from build123d import *

# Parameters (mm, degrees)
SKETCH1_W           = 76.33
SKETCH1_H           = 76.33
BOSS_EXTRUDE1_DEPTH = 76.33
SKETCH2_R           = 35
BOSS_EXTRUDE2_DEPTH = 36.82
CHAMFER1_SIZE       = 2.5
CUT_EXTRUDE1_REACH  = 1889.491
CUT_EXTRUDE2_DEPTH  = 0.5


with BuildPart() as part:
    # Sketch1 → Boss-Extrude1 (new body)
    with BuildSketch(Plane.ZY.offset(-1848.740517551)):
        Rectangle(SKETCH1_W, SKETCH1_H)
    extrude(amount=BOSS_EXTRUDE1_DEPTH)

    # Sketch2 → Boss-Extrude2 (add)
    with BuildSketch(Plane(origin=(1848.740517551, 0, 0), x_dir=(0, 0, -1), z_dir=(1, 0, 0))):
        with Locations(Location((0, 0, 0), (0, 0, 90))):
            Circle(SKETCH2_R)
    extrude(amount=BOSS_EXTRUDE2_DEPTH)

    # Chamfer1
    chamfer1_edges = [part.edges().sort_by_distance(p)[0] for p in [
        (1772.410517551, -38.165, 0),
        (1772.410517551, 0, -38.165),
        (1772.410517551, 38.165, 0),
        (1848.740517551, 0, -38.165),
        (1848.740517551, -38.165, 0),
        (1848.740517551, 0, 38.165),
        (1848.740517551, 38.165, 0),
        (1772.410517551, 0, 38.165),
        (1810.575517551, 38.165, -38.165),
        (1810.575517551, -38.165, -38.165),
        (1810.575517551, -38.165, 38.165),
        (1810.575517551, 38.165, 38.165),
    ]]
    chamfer(chamfer1_edges, length=CHAMFER1_SIZE)

    # Sketch3 → Cut-Extrude1 (cut, up to next)
    with BuildSketch(Plane(origin=(0, 0, -38.165), x_dir=(-1, 0, 0), z_dir=(0, 0, -1)), mode=Mode.PRIVATE) as cut_extrude1_sk1:
        with BuildLine():
            ThreePointArc((-1791.865517551, 0), (-1797.345549675, 13.229967876), (-1810.575517551, 18.71))
            Line((-1810.575517551, 18.71), (-1810.575517551, -18.71))
            ThreePointArc((-1810.575517551, -18.71), (-1797.345549675, -13.229967876), (-1791.865517551, 0))
        make_face()
    cut_extrude1_tool1 = extrude(cut_extrude1_sk1.sketch, amount=-CUT_EXTRUDE1_REACH, mode=Mode.PRIVATE) & part.part
    # Sketch3 → Cut-Extrude1 (cut, up to next)
    with BuildSketch(Plane(origin=(0, 0, -38.165), x_dir=(-1, 0, 0), z_dir=(0, 0, -1)), mode=Mode.PRIVATE) as cut_extrude1_sk2:
        with BuildLine():
            Line((-1810.575517551, -18.71), (-1810.575517551, 18.71))
            ThreePointArc((-1810.575517551, 18.71), (-1829.285517551, 0), (-1810.575517551, -18.71))
        make_face()
    cut_extrude1_tool2 = extrude(cut_extrude1_sk2.sketch, amount=-CUT_EXTRUDE1_REACH, mode=Mode.PRIVATE) & part.part
    # Sketch3 → Cut-Extrude1 (cut, up to next)
    with BuildSketch(Plane(origin=(0, 0, -38.165), x_dir=(-1, 0, 0), z_dir=(0, 0, -1)), mode=Mode.PRIVATE) as cut_extrude1_sk3:
        with BuildLine():
            ThreePointArc((-1791.865517551, 0), (-1797.345549675, 13.229967876), (-1810.575517551, 18.71))
            Line((-1810.575517551, 18.71), (-1810.575517551, -18.71))
            ThreePointArc((-1810.575517551, -18.71), (-1797.345549675, -13.229967876), (-1791.865517551, 0))
        make_face()
    cut_extrude1_tool3 = extrude(cut_extrude1_sk3.sketch, amount=-CUT_EXTRUDE1_REACH, mode=Mode.PRIVATE) & part.part
    # Sketch3 → Cut-Extrude1 (cut, up to next)
    with BuildSketch(Plane(origin=(0, 0, -38.165), x_dir=(-1, 0, 0), z_dir=(0, 0, -1)), mode=Mode.PRIVATE) as cut_extrude1_sk4:
        with BuildLine():
            Line((-1810.575517551, -18.71), (-1810.575517551, 18.71))
            ThreePointArc((-1810.575517551, 18.71), (-1829.285517551, 0), (-1810.575517551, -18.71))
        make_face()
    cut_extrude1_tool4 = extrude(cut_extrude1_sk4.sketch, amount=-CUT_EXTRUDE1_REACH, mode=Mode.PRIVATE) & part.part
    add(cut_extrude1_tool1.solids().sort_by_distance((1802.634747, 0, -38.165))[0], mode=Mode.SUBTRACT)
    add(cut_extrude1_tool2.solids().sort_by_distance((1818.516288, 0, -38.165))[0], mode=Mode.SUBTRACT)
    add(cut_extrude1_tool3.solids().sort_by_distance((1802.634747, 0, -38.165))[0], mode=Mode.SUBTRACT)
    add(cut_extrude1_tool4.solids().sort_by_distance((1818.516288, 0, -38.165))[0], mode=Mode.SUBTRACT)

    # Sketch5 → Cut-Extrude2 (cut)
    with BuildSketch(Plane(origin=(0, 38.165, 0), x_dir=(1, 0, 0), z_dir=(0, 1, 0))):
        with BuildLine():
            Line((1788.358917551, -32.3946), (1832.792217551, -32.3946))
            add(Edge.make_bspline(
                [(1832.792217551, -32.3946), (1833.466855861, -32.3946), (1834.834608919, -32.253703608), (1837.339344692, -31.462150857), (1840.043615022, -29.624585418), (1841.881171353, -26.92029094), (1842.672721425, -24.415524634), (1842.813617551, -23.047748692), (1842.813617551, -22.3731)],
                knots=[0.555555556, 0.555555556, 0.555555556, 0.555555556, 0.569444444, 0.583333333, 0.611111111, 0.638888889, 0.652777778, 0.666666667, 0.666666667, 0.666666667, 0.666666667], degree=3))
            Line((1842.813617551, -22.3731), (1842.813617551, 22.373))
            add(Edge.make_bspline(
                [(1842.813617551, 22.373), (1842.813617551, 23.047629093), (1842.672720901, 24.415360154), (1841.881169744, 26.92007933), (1840.043614741, 29.624353237), (1837.339347144, 31.46193401), (1834.834610984, 32.25350014), (1833.466856595, 32.3944), (1832.792217551, 32.3944)],
                knots=[0.777777778, 0.777777778, 0.777777778, 0.777777778, 0.805555556, 0.833333333, 0.888888889, 0.944444444, 0.972222222, 1, 1, 1, 1], degree=3))
            Line((1832.792217551, 32.3944), (1788.358917551, 32.3944))
            add(Edge.make_bspline(
                [(1788.358917551, 32.3944), (1787.684278508, 32.3944), (1786.316524118, 32.25350014), (1783.811787958, 31.46193401), (1781.107520362, 29.624353237), (1779.269965358, 26.92007933), (1778.478414202, 24.415360154), (1778.337517551, 23.047629093), (1778.337517551, 22.373)],
                knots=[0.111111111, 0.111111111, 0.111111111, 0.111111111, 0.125, 0.138888889, 0.166666667, 0.194444444, 0.208333333, 0.222222222, 0.222222222, 0.222222222, 0.222222222], degree=3))
            Line((1778.337517551, 22.373), (1778.337517551, -22.3731))
            add(Edge.make_bspline(
                [(1778.337517551, -22.3731), (1778.337517551, -23.047748692), (1778.478413677, -24.415524634), (1779.269963749, -26.92029094), (1781.107520081, -29.624585418), (1783.81179041, -31.462150857), (1786.316526183, -32.253703608), (1787.684279242, -32.3946), (1788.358917551, -32.3946)],
                knots=[0.333333333, 0.333333333, 0.333333333, 0.333333333, 0.347222222, 0.361111111, 0.388888889, 0.416666667, 0.430555556, 0.444444444, 0.444444444, 0.444444444, 0.444444444], degree=3))
        make_face()
        with BuildLine():
            Line((1788.358917551, -31.3946), (1832.792217551, -31.3946))
            add(Edge.make_bspline(
                [(1832.792217551, -31.3946), (1833.399248628, -31.3946), (1834.630365029, -31.267771469), (1836.881569909, -30.556358134), (1839.319622864, -28.900598899), (1840.975375901, -26.462522118), (1841.686788747, -24.211284373), (1841.813617551, -22.980142574), (1841.813617551, -22.3731)],
                knots=[0.555555556, 0.555555556, 0.555555556, 0.555555556, 0.569444444, 0.583333333, 0.611111111, 0.638888889, 0.652777778, 0.666666667, 0.666666667, 0.666666667, 0.666666667], degree=3))
            Line((1841.813617551, -22.3731), (1841.813617551, 22.373))
            add(Edge.make_bspline(
                [(1841.813617551, 22.373), (1841.813617551, 22.980021237), (1841.686789271, 24.211113504), (1840.975377513, 26.462304848), (1839.319623121, 28.900367756), (1836.881567526, 30.556143835), (1834.630362845, 31.267568666), (1833.399248157, 31.3944), (1832.792217551, 31.3944)],
                knots=[0.777777778, 0.777777778, 0.777777778, 0.777777778, 0.805555556, 0.833333333, 0.888888889, 0.944444444, 0.972222222, 1, 1, 1, 1], degree=3))
            Line((1832.792217551, 31.3944), (1788.358917551, 31.3944))
            add(Edge.make_bspline(
                [(1788.358917551, 31.3944), (1787.751886946, 31.3944), (1786.520772257, 31.267568666), (1784.269567577, 30.556143835), (1781.831511982, 28.900367756), (1780.175757589, 26.462304848), (1779.464345832, 24.211113504), (1779.337517551, 22.980021237), (1779.337517551, 22.373)],
                knots=[0.111111111, 0.111111111, 0.111111111, 0.111111111, 0.125, 0.138888889, 0.166666667, 0.194444444, 0.208333333, 0.222222222, 0.222222222, 0.222222222, 0.222222222], degree=3))
            Line((1779.337517551, 22.373), (1779.337517551, -22.3731))
            add(Edge.make_bspline(
                [(1779.337517551, -22.3731), (1779.337517551, -22.980142574), (1779.464346356, -24.211284373), (1780.175759201, -26.462522118), (1781.831512239, -28.900598899), (1784.269565194, -30.556358134), (1786.520770074, -31.267771469), (1787.751886474, -31.3946), (1788.358917551, -31.3946)],
                knots=[0.333333333, 0.333333333, 0.333333333, 0.333333333, 0.347222222, 0.361111111, 0.388888889, 0.416666667, 0.430555556, 0.444444444, 0.444444444, 0.444444444, 0.444444444], degree=3))
        make_face(mode=Mode.SUBTRACT)
    extrude(amount=-CUT_EXTRUDE2_DEPTH, mode=Mode.SUBTRACT)


solid = part.part
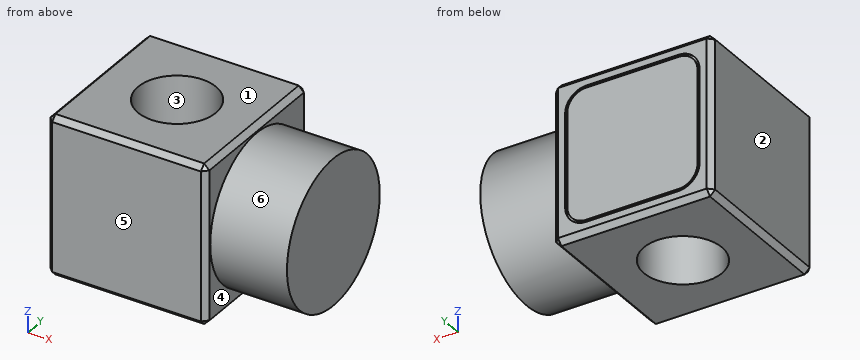
Here's how the part is built. I have some questions about the finished solid (model axes, mm). Face numbers are marked on the shaded views. A direction names the side the tool comes from. Round coordinates to 2 decimals unless told otherwise and drop trailing zeros. Write each loop counter-clockwise with the first axis right and the second up, starting at its lowest first coordinate (ties: lowest second). Pieces come first, ordered by that corner, then holes. Notation, with made-up numbers: (54.25, 49) -> (69.25, 49) arc R22 cw to (69.25, 69) -> close; hole circle Ø9 at (-15, 16.5). An arc over 180 degrees is marked (long way). One line per item, written item: value.
1) Suppose I cut it at C-C on x = 1800. List the corners of the cut face in (y, z) for me (3 decimals).
Filled sheet:
outline: (-38.165, -35.665) -> (-35.665, -38.165) -> (-15.434, -38.165) -> (-15.434, 38.165) -> (-35.665, 38.165) -> (-38.165, 35.665) -> close; (15.434, -38.165) -> (35.665, -38.165) -> (38.165, -35.665) -> (38.165, -32.394) -> (37.665, -32.394) -> (37.665, -31.394) -> (38.165, -31.394) -> (38.165, 31.395) -> (37.665, 31.395) -> (37.665, 32.395) -> (38.165, 32.395) -> (38.165, 35.665) -> (35.665, 38.165) -> (15.434, 38.165) -> close
2) Suppose I cut it at D-D on y = 14. List the corners of the cut face in (x, z) for me (3 decimals).
Filled sheet:
outline: (1772.411, -35.665) -> (1774.911, -38.165) -> (1798.163, -38.165) -> (1798.163, 38.165) -> (1774.911, 38.165) -> (1772.411, 35.665) -> close; (1822.988, -38.165) -> (1846.241, -38.165) -> (1848.741, -35.665) -> (1848.741, -32.078) -> (1885.561, -32.078) -> (1885.561, 32.078) -> (1848.741, 32.078) -> (1848.741, 35.665) -> (1846.241, 38.165) -> (1822.988, 38.165) -> close
3) We'd pull the mould along X, two halves only. Please class the marked faces 1, 2, 3 and 4: released by +X, released by -X, zero draft, split by the parting line, or undercut.
Filled sheet:
face 1: zero draft
face 2: released by -X
face 3: undercut
face 4: released by +X
4) For the marked faces 5 and 6, which set-ups out of +Z, -Z, +X, -X, +Y, -Y let a thin tool reach every point of the face, with its end or its side?
Filled sheet:
face 5: +Z, -Z, +X, -X, -Y
face 6: +X
5) Suppose I cut it at A-A on y = 0. List the corners of the cut face in (x, z) for me (3 decimals), plus the area to 3 significant figures.
Filled sheet:
outline: (1772.411, -35.665) -> (1774.911, -38.165) -> (1791.866, -38.165) -> (1791.866, 38.165) -> (1774.911, 38.165) -> (1772.411, 35.665) -> close; (1829.286, -38.165) -> (1846.241, -38.165) -> (1848.741, -35.665) -> (1848.741, -35) -> (1885.561, -35) -> (1885.561, 35) -> (1848.741, 35) -> (1848.741, 35.665) -> (1846.241, 38.165) -> (1829.286, 38.165) -> close
area: 5,530 mm2
6) Suppose I cut it at B-B on z = -8. List the corners of the cut face in (x, y) for me (3 decimals).
Filled sheet:
outline: (1772.411, -35.665) -> (1774.911, -38.165) -> (1846.241, -38.165) -> (1848.741, -35.665) -> (1848.741, -34.073) -> (1885.561, -34.073) -> (1885.561, 34.073) -> (1848.741, 34.073) -> (1848.741, 35.665) -> (1846.241, 38.165) -> (1842.814, 38.165) -> (1842.814, 37.665) -> (1841.814, 37.665) -> (1841.814, 38.165) -> (1779.338, 38.165) -> (1779.338, 37.665) -> (1778.338, 37.665) -> (1778.338, 38.165) -> (1774.911, 38.165) -> (1772.411, 35.665) -> close; hole circle Ø37.42 at (1810.576, 0)
7) I'm going to push flat-ended pins straight in: pin 1 Ø10 at (x, y) = (1866.5, 25.5) entering from +Z; pin 2 Ø0.6 at (x, y) = (1819, 38) entering from -Z; pin 3 Ø0.6 at (y, z) = (38, 10.5) entering from -X. Where does each tip first touch, or does it pass through?
Filled sheet:
pin 1: stops at z = 28.37
pin 2: stops at z = -36.13
pin 3: stops at x = 1774.45
8) If I drill on line 1 (X direction, y = 0, z = -15); line 2 (Y direction, x = 1808, z = -10) (3 decimals); line 3 (X direction, y = 8.5, z = -20), over which ranges is the centre line in solid material (lowest first)? Write a range as [from, to].
Filled sheet:
line 1: x = [1772.41, 1791.87], [1829.29, 1885.56]
line 2: y = [-38.165, -18.532], [18.532, 38.165]
line 3: x = [1772.41, 1793.91], [1827.24, 1885.56]
